Read the model definition and answer for the solid it produces. Units are mm, in the model's axes. A direction names the side the tool comes from. Round coordinates to 2 decimals unless told otherwise and drop trailing zeros. Order: outer loops, then holes, each group sorted by start corner. A loop starts at its lowest first (then second) coordinate and runs counter-clockwise, first axis right, second up.
from build123d import *

# Parameters (mm, degrees)
CROQUIS1_W              = 60
CROQUIS1_H              = 35
CROQUIS1_W_2            = 30
CROQUIS1_H_2            = 15
SALIENTE_EXTRUIR1_DEPTH = 5
CHAFL_N2_SIZE           = 4
CHAFL_N2_SIZE2          = 5
CHAFL_N2_PART_2_SIZE    = 4
CHAFL_N2_PART_2_SIZE2   = 5
CHAFL_N3_SIZE           = 5
CHAFL_N3_SIZE2          = 4
CHAFL_N3_PART_2_SIZE    = 5
CHAFL_N3_PART_2_SIZE2   = 4
CHAFL_N1_SIZE           = 3
CROQUIS2_W              = 60
CROQUIS2_H              = 8
SALIENTE_EXTRUIR2_DEPTH = 20
CORTAR_EXTRUIR1_DEPTH   = 9
CROQUIS4_W              = 3
CROQUIS4_H              = 35
SALIENTE_EXTRUIR3_DEPTH = 15
CORTAR_EXTRUIR2_DEPTH   = 10
REDONDEO1_R             = 10


with BuildPart() as part:
    # Croquis1 → Saliente-Extruir1 (new body)
    with BuildSketch(Plane.XY):
        with Locations((30, 17.5)):
            Rectangle(CROQUIS1_W, CROQUIS1_H)
        with Locations((30, 17.5)):
            Rectangle(CROQUIS1_W_2, CROQUIS1_H_2, mode=Mode.SUBTRACT)
    extrude(amount=SALIENTE_EXTRUIR1_DEPTH)

    # Chaflán2
    chafl_n2_edges = [part.edges().sort_by_distance(p)[0] for p in [
        (15, 25, 2.5),
    ]]
    chafl_n2_side = [part.faces().sort_by_distance(p)[0] for p in [
        (15, 17.5, 2.5),
    ]]
    chamfer(chafl_n2_edges, length=CHAFL_N2_SIZE, length2=CHAFL_N2_SIZE2, reference=chafl_n2_side[0])

    # Chaflán2 part 2
    chafl_n2_part_2_edges = [part.edges().sort_by_distance(p)[0] for p in [
        (45, 10, 2.5),
    ]]
    chafl_n2_part_2_side = [part.faces().sort_by_distance(p)[0] for p in [
        (45, 17.5, 2.5),
    ]]
    chamfer(chafl_n2_part_2_edges, length=CHAFL_N2_PART_2_SIZE, length2=CHAFL_N2_PART_2_SIZE2, reference=chafl_n2_part_2_side[0])

    # Chaflán3
    chafl_n3_edges = [part.edges().sort_by_distance(p)[0] for p in [
        (15, 10, 2.5),
    ]]
    chafl_n3_side = [part.faces().sort_by_distance(p)[0] for p in [
        (27.5, 10, 2.5),
    ]]
    chamfer(chafl_n3_edges, length=CHAFL_N3_SIZE, length2=CHAFL_N3_SIZE2, reference=chafl_n3_side[0])

    # Chaflán3 part 2
    chafl_n3_part_2_edges = [part.edges().sort_by_distance(p)[0] for p in [
        (45, 25, 2.5),
    ]]
    chafl_n3_part_2_side = [part.faces().sort_by_distance(p)[0] for p in [
        (32.5, 25, 2.5),
    ]]
    chamfer(chafl_n3_part_2_edges, length=CHAFL_N3_PART_2_SIZE, length2=CHAFL_N3_PART_2_SIZE2, reference=chafl_n3_part_2_side[0])

    # Chaflán1
    chafl_n1_edges = [part.edges().sort_by_distance(p)[0] for p in [
        (45, 17.5, 5),
        (15, 17.5, 5),
        (42.5, 12, 5),
        (17.5, 23, 5),
        (30, 25, 5),
        (30, 10, 5),
        (42.5, 23, 5),
        (17.5, 12, 5),
    ]]
    chamfer(chafl_n1_edges, length=CHAFL_N1_SIZE)

    # Croquis2 → Saliente-Extruir2 (add)
    with BuildSketch(Plane(origin=(0, 0, 0), x_dir=(-1, 0, 0), z_dir=(0, 0, -1))):
        with Locations((-30, 39)):
            Rectangle(CROQUIS2_W, CROQUIS2_H)
    extrude(amount=-SALIENTE_EXTRUIR2_DEPTH)

    # Croquis3 → Cortar-Extruir1 (cut, through all)
    with BuildSketch(Plane.XZ.offset(-35)):
        with BuildLine():
            Line((9.955719163, 11.839406388), (11, 13))
            Line((11, 13), (13, 13))
            Line((13, 13), (14.044280837, 11.839406388))
            ThreePointArc((14.044280837, 11.839406388), (12, 7.25), (9.955719163, 11.839406388))
        make_face()
        with BuildLine():
            Line((47.955719163, 11.839406388), (49, 13))
            Line((49, 13), (51, 13))
            Line((51, 13), (52.044280837, 11.839406388))
            ThreePointArc((52.044280837, 11.839406388), (50, 7.25), (47.955719163, 11.839406388))
        make_face()
    extrude(amount=-CORTAR_EXTRUIR1_DEPTH, mode=Mode.SUBTRACT)

    # Croquis4 → Saliente-Extruir3 (add)
    with BuildSketch(Plane.XY.offset(5)):
        with Locations((1.5, 17.5)):
            Rectangle(CROQUIS4_W, CROQUIS4_H)
    extrude(amount=SALIENTE_EXTRUIR3_DEPTH)

    # Croquis5 → Cortar-Extruir2 (cut)
    with BuildSketch(Plane.ZY):
        with BuildLine():
            Line((12.886683465, 12.445791337), (14.1, 11.6))
            Line((14.1, 11.6), (14.1, 9.6))
            Line((14.1, 9.6), (12.886683465, 8.754208663))
            ThreePointArc((12.886683465, 8.754208663), (9.35, 10.6), (12.886683465, 12.445791337))
        make_face()
    extrude(amount=-CORTAR_EXTRUIR2_DEPTH, mode=Mode.SUBTRACT)

    # Redondeo1
    redondeo1_edges = [part.edges().sort_by_distance(p)[0] for p in [
        (1.5, 0, 20),
    ]]
    fillet(redondeo1_edges, radius=REDONDEO1_R)


solid = part.part
Q1. Straight lines are drawn through the part: probe 1 along X at (y, z) = (38.5, 10); probe 2 along Z at (x, y) = (50, 37.25); probe 3 along Z at (x, y) = (2, 10.6). For each, find the intervals that lie inside material, in ascending order.
Outcome:
probe 1: x = 0 to 9.25, 14.75 to 47.25, 52.75 to 60
probe 2: z = 0 to 7.25, 13 to 20
probe 3: z = 0 to 9.35, 14.1 to 20
Q2. Flat-ended cylindrical pins translate along their axes: pin 1 (7 mm diameter, centred on x = 50, z = 10, fed in from +Y); pin 2 (7 mm diameter, centred on x = 12, z = 10, fed in from -Y); pin 3 (8 mm diameter, centred on x = 52, y = 21.5, fed in from +Z). Find the tip coordinate at first contact, or state that the pin passes through.
Outcome:
pin 1: stops at y = 43
pin 2: stops at y = 35
pin 3: stops at z = 5
Q3. For a pull along Z with two mould halves and no side action, classify faces 4 (the face through (16.446, 10.895, 3.521)), 5 (the face through (13.515, 38.944, 12.428)), 6 (the face through (0, 21, 10)), 7 (the face through (30, 27, 0)) as released by +Z, released by -Z, zero draft, split by the parting line, or undercut.
Outcome:
face 4: released by +Z
face 5: undercut
face 6: zero draft
face 7: released by -Z
Q4. A cutting plane is placed at B-B, the plane z = 6. Give the vertices of the cut face in (x, y).
Outcome:
outline: (0, 0) - (3, 0) - (3, 35) - (60, 35) - (60, 43) - (0, 43) - close
Q5. A cutting plane is placed at C-C, the plane x = 50. Give the vertices of the cut face in (y, z), plus the area to 3 significant figures.
Outcome:
outline: (0, 0) - (43, 0) - (43, 7.25) - (35, 7.25) - (35, 5) - (0, 5) - close; (35, 13) - (43, 13) - (43, 20) - (35, 20) - close
area: 289 mm2
Q6. A cutting plane is placed at D-D, the plane y = 3.5. Give the vertices of the cut face in (x, z).
Outcome:
outline: (0, 0) - (60, 0) - (60, 5) - (3, 5) - (3, 17.6) - (0, 17.6) - close
Q7. For faces 1 (the face through (3, 17, 12)), 2 (the face through (43.65, 10.97, 3.52)), 3 (the face through (48.47, 38.94, 12.41)), determine the directions among +Z, -Z, +X, -X, +Y, -Y from which every point of the face is accessible in a straight line to the end or side of a thin tool.
Outcome:
face 1: +Z, +X, -Y
face 2: +Z
face 3: +Y, -Y
Q8. A cutting plane is placed at A-A, the plane x = 22.5. Give the vertices of the cut face in (y, z), plus the area to 3 significant figures.
Outcome:
outline: (0, 0) - (10, 0) - (10, 2) - (7, 5) - (0, 5) - close; (25, 0) - (43, 0) - (43, 20) - (35, 20) - (35, 5) - (28, 5) - (25, 2) - close
area: 251 mm2
